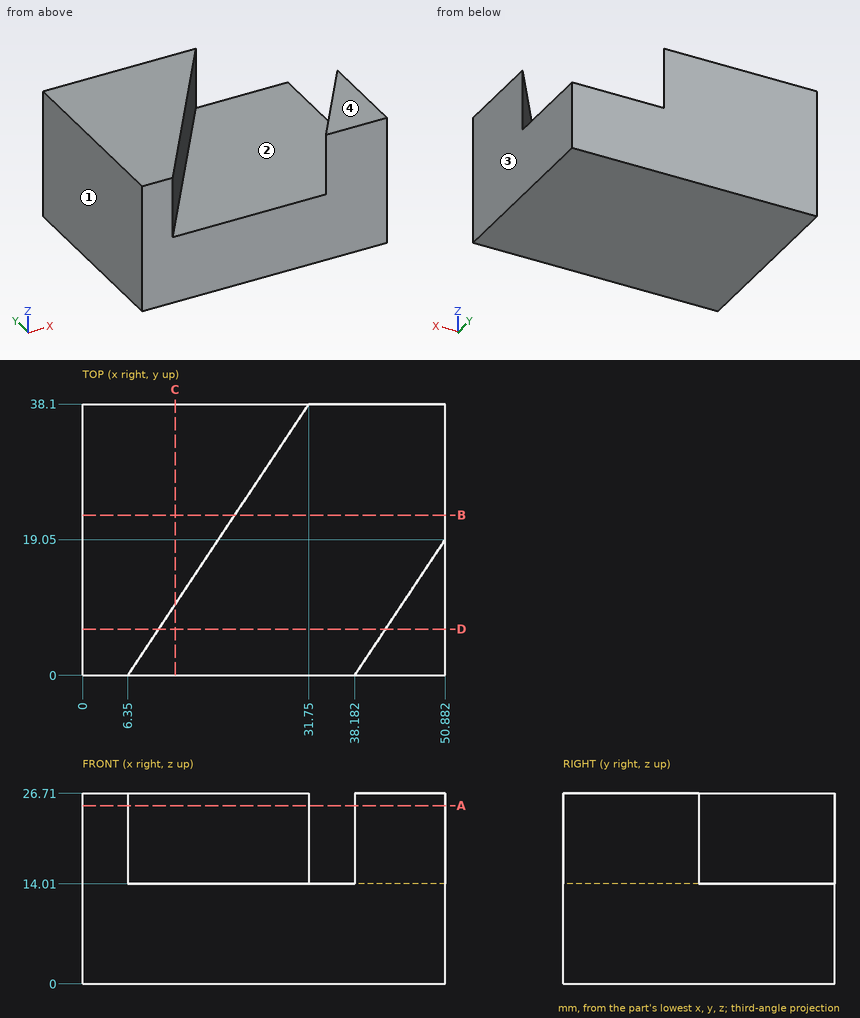
Job drawing, mm, ordinate dimensions from the low corner. One solid piece. Give positions to 0.01 mm unless a question says otherwise; leave off trailing zeros. Loops run counter-clockwise (first coordinate to the right, second up) from the corner with the lowest first, then second, coordinate; pieces in that order, holes last. Notation, with made-up numbers: (-6, 68.5) -> (32, 68.5) arc R25 ccw to (32, 92.5) -> close; hole circle Ø4 at (51, 63.5). An arc over 180 degrees is marked (long way). Use a Markdown table: item, result. Add a question column.
(1) Slice it at B-B on y = 22.5. List the corners of the cut face in (x, z), and give its area (3 significant figures).
(2) Slice it at A-A on z = 25. List the corners of the cut face in (x, y).
(3) Slice it at C-C on x = 13. List the corners of the cut face in (y, z) (1 decimal).
(4) Slice it at D-D on y = 6.5. List the corners of the cut face in (x, z) (1 decimal), and give its area (3 significant figures).
(5) Wall check: line 1 along Z through (x, y) = (39, 8.5); line 2 along X through (y, z) = (10.5, 23.25); line 3 along X through (y, z) = (4.5, 20.25). Give the ranges that are in metal, low to high.
(6) Mould opens along X. For the marked faces 1, 2, 3 and 4 say: +X half, -X half, draft (parallel to the pull), parting line (faces both ways), or undercut.
(7) Drop flat-ended pins along their axis: pin 1 Ø10 at (x, z) = (38.5, 22.5) entering from +Y (1 decimal); pin 2 Ø1 at (y, z) = (12, 19) entering from -X; pin 3 Ø8 at (x, y) = (43, 28.5) entering from +Z. Give the stop position or say it passes through.
Filled sheet:
| question | item | result |
|---|---|---|
| 1 | outline | (0, 0) -> (50.88, 0) -> (50.88, 14.01) -> (21.35, 14.01) -> (21.35, 26.71) -> (0, 26.71) -> close |
| 1 | area | 984 mm2 |
| 2 | outline | (0, 0) -> (6.35, 0) -> (31.75, 38.1) -> (0, 38.1) -> close; (38.18, 0) -> (50.88, 0) -> (50.88, 19.05) -> close |
| 3 | outline | (0, 0) -> (38.1, 0) -> (38.1, 26.7) -> (10, 26.7) -> (10, 14) -> (0, 14) -> close |
| 4 | outline | (0, 0) -> (50.9, 0) -> (50.9, 26.7) -> (42.5, 26.7) -> (42.5, 14) -> (10.7, 14) -> (10.7, 26.7) -> (0, 26.7) -> close |
| 4 | area | 955 mm2 |
| 5 | line 1 | 0 to 14.01 |
| 5 | line 2 | 0 to 13.35, 45.18 to 50.88 |
| 5 | line 3 | 0 to 9.35, 41.18 to 50.88 |
| 6 | face 1 | -X half |
| 6 | face 2 | undercut |
| 6 | face 3 | +X half |
| 6 | face 4 | draft |
| 7 | pin 1 | y = 8 |
| 7 | pin 2 | x = 0 |
| 7 | pin 3 | z = 14.01 |
